The listing builds one solid part. Answer for the finished solid, in the listing's coordinates (mm). Round coordinates to 2 decimals unless told otherwise and drop trailing zeros. Order: outer loops, then holes, each group sorted by start corner. A loop starts at its lowest first (then second) coordinate and runs counter-clockwise, first axis right, second up. Notation, with made-up numbers: M -33,4.25 L -28,4.25 A23 ccw -28,42.25 Z; hole C 9.5,87.5 d9. An arc over 180 degrees is marked long. Write item = value, one per line. Start each with the question number.
(1) A cutting plane is placed at B-B, the plane y = 2.5. Determine the outline of the cut face in (x, z).
(2) A cutting plane is placed at C-C, the plane z = 21. Determine the outline of the cut face in (x, y), and give its area (3 significant figures).
(3) A cutting plane is placed at D-D, the plane x = -41. Determine the outline of the cut face in (y, z).
(4) Straight lines are drawn through the part: probe 1 along X at (y, z) = (2.15, 13.75); probe 2 along X at (y, z) = (2.95, 16.5); probe 3 along Z at (x, y) = (-17, 0.45). For each, find the intervals that lie inside material, in ascending order. Write a range as from..to.
(5) A cutting plane is placed at A-A, the plane x = -18. Determine the outline of the cut face in (y, z).
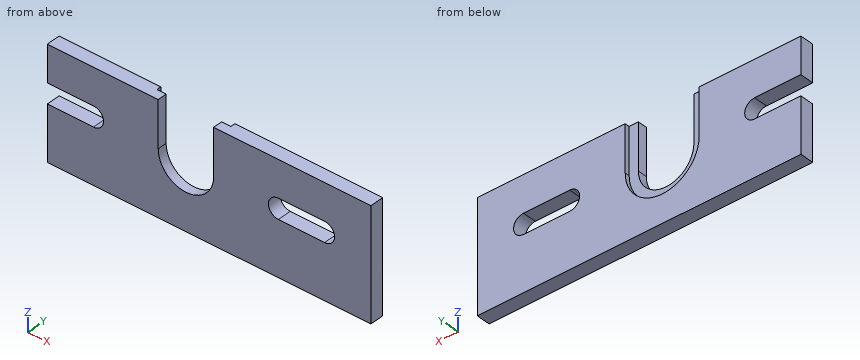
Autodesk Inventor part; units mm, degrees
ref_plane "YZ Plane" through (0, 0, 0) normal (1, 0, 0) x (0, 1, 0)
ref_plane "XZ Plane" through (0, 0, 0) normal (0, 1, 0) x (-1, 0, 0)
ref_plane "XY Plane" through (0, 0, 0) normal (0, 0, 1) x (1, 0, 0)
sketch "Sketch1" plane through (0, 0, 0) normal (0, 1, 0) x (-1, 0, 0)
  line L0 (0, 0) -> (70, 0)
  line L1 (70, 0) -> (70, 24)
  line L2 (70, 24) -> (0, 24)
  line L3 (0, 24) -> (0, 0)
  dimension "d0" = 70
  dimension "d1" = 24
extrude "Extrusion1" add sketch "Sketch1" along normal blind 3
sketch "Sketch2" plane through (0, 3, 0) normal (0, 1, 0) x (1, 0, 0)
  line L0 (-70, 0) -> (-70, -24)
  line L1 (-70, -24) -> (0, -24)
  arc A0 (-32, -14) -> (-48, -14) centre (-40, -14) ccw
  line L2 (-32, -14) -> (-32, -24)
  line L3 (-48, -14) -> (-48, -24)
  dimension "d5" = 16
  dimension "d6" = 10
  dimension "d8" = 30
extrude "Extrusion2" cut sketch "Sketch2" against normal blind 1
sketch "Sketch3" plane through (0, 2, 0) normal (0, 1, 0) x (1, 0, 0)
  arc A0 (-32, -14) -> (-48, -14) centre (-40, -14) ccw
  line L0 (-32, -24) -> (-48, -24)
  arc A1 (-34, -14) -> (-46, -14) centre (-40, -14) ccw
  line L1 (-46, -14) -> (-46, -24)
  line L2 (-34, -14) -> (-34, -24)
  point P0 (0, 0)
  dimension "d11" = 12
extrude "Extrusion3" cut sketch "Sketch3" against normal blind 2
sketch "Sketch4" plane through (0, 3, 0) normal (0, 1, 0) x (1, 0, 0)
  line L0 (-32, -24) -> (0, -24)
  line L1 (0, -24) -> (0, 0)
  line L2 (-70, 0) -> (-70, -24)
  arc A0 (-32, -14) -> (-48, -14) centre (-40, -14) ccw
  line L3 (-70, -14) -> (-60, -14) construction
  line L4 (-70, -16.15) -> (-60, -16.15)
  line L5 (-60, -11.85) -> (-70, -11.85)
  arc A1 (-70, -11.85) -> (-70, -16.15) centre (-70, -14) ccw
  arc A2 (-60, -16.15) -> (-60, -11.85) centre (-60, -14) ccw
  line L6 (-20, -14) -> (-10, -14) construction
  line L7 (-20, -16.15) -> (-10, -16.15)
  line L8 (-10, -11.85) -> (-20, -11.85)
  arc A3 (-20, -11.85) -> (-20, -16.15) centre (-20, -14) ccw
  arc A4 (-10, -16.15) -> (-10, -11.85) centre (-10, -14) ccw
  point P0 (-65, -14)
  point P1 (-15, -14)
  dimension "d14" = 5
  dimension "d15" = 4.3
  dimension "d16" = 5
  dimension "d17" = 5
  dimension "d18" = 4.3
  dimension "d19" = 15
extrude "Extrusion4" cut sketch "Sketch4" against normal blind 3
properties part number "JHeadMount" material "Aluminum 6061"
Reported:
q1.outline = M -70,0 L 0,0 L 0,24 L -32,24 L -32,14 A8 cw -48,14 L -48,24 L -70,24 L -70,16.15 L -60,16.15 A2.15 cw -60,11.85 L -70,11.85 Z; hole M -20,11.85 L -10,11.85 A2.15 ccw -10,16.15 L -20,16.15 A2.15 ccw Z
q2.outline = M -70,0 L -46,0 L -46,2 L -48,2 L -48,3 L -70,3 Z; M -34,0 L 0,0 L 0,3 L -32,3 L -32,2 L -34,2 Z
q2.area = 170 mm²
q3.outline = M 0,0 L 3,0 L 3,6.06 L 2,6.06 L 2,8.08 L 0,8.08 Z
q4.probe_1 = -57.86..-48, -32..-22.14, -7.86..0
q4.probe_2 = -70..-48, -32..0
q4.probe_3 = 0..11.85, 16.15..24
q5.outline = M 0,0 L 3,0 L 3,11.85 L 0,11.85 Z; M 0,16.15 L 3,16.15 L 3,24 L 0,24 Z
